```python
from build123d import *

# Parameters (mm, degrees)
SKETCH_W      = 100
SKETCH_H      = 80
SKETCH_R      = 1.75
PAD_DEPTH     = 4.5
CHAMFER_SIZE  = 1.5
SKETCH001_W   = 100
SKETCH001_H   = 80
SKETCH001_W_2 = 97
SKETCH001_H_2 = 77
PAD001_DEPTH  = 45
SKETCH002_W   = 100
SKETCH002_H   = 80
SKETCH002_R   = 1.75
PAD002_DEPTH  = 3.5


with BuildPart() as part:
    # Sketch → Pad (new body)
    with BuildSketch(Plane.XY):
        with Locations((-14.266246, -4.330319)):
            Rectangle(SKETCH_W, SKETCH_H)
        with Locations((-59.499317, 30.08403)):
            Circle(SKETCH_R, mode=Mode.SUBTRACT)
        with Locations((28.500683, 29.937424)):
            Circle(SKETCH_R, mode=Mode.SUBTRACT)
        with Locations((-59.584126, -34.915915)):
            Circle(SKETCH_R, mode=Mode.SUBTRACT)
        with Locations((28.415874, -35.062521)):
            Circle(SKETCH_R, mode=Mode.SUBTRACT)
    extrude(amount=PAD_DEPTH)

    # Chamfer
    chamfer_edges = [part.edges().sort_by_distance(p)[0] for p in [
        (-61.334126, -34.915915, 0),
        (26.665874, -35.062521, 0),
        (26.750683, 29.937424, 0),
        (-61.249317, 30.08403, 0),
    ]]
    chamfer(chamfer_edges, length=CHAMFER_SIZE)

    # Sketch001 (on Face3 of Chamfer) → Pad001 (join)
    with BuildSketch(Plane.XY.offset(4.5)):
        with Locations((-14.266246, -4.330319)):
            Rectangle(SKETCH001_W, SKETCH001_H)
        with Locations((-14.266246, -4.330319)):
            Rectangle(SKETCH001_W_2, SKETCH001_H_2, mode=Mode.SUBTRACT)
    extrude(amount=PAD001_DEPTH)

    # Sketch002 (on Face19 of Pad001) → Pad002 (join)
    with BuildSketch(Plane.XY.offset(49.5)):
        with Locations((-14.266246, -4.330319)):
            Rectangle(SKETCH002_W, SKETCH002_H)
        with Locations((-59.499317, 30.08403)):
            Circle(SKETCH002_R, mode=Mode.SUBTRACT)
        with Locations((-59.584126, -34.915915)):
            Circle(SKETCH002_R, mode=Mode.SUBTRACT)
        with Locations((28.500683, 29.937424)):
            Circle(SKETCH002_R, mode=Mode.SUBTRACT)
        with Locations((28.415874, -35.062521)):
            Circle(SKETCH002_R, mode=Mode.SUBTRACT)
    extrude(amount=PAD002_DEPTH)


solid = part.part
```
Here's how the part is built. I have some questions about the finished solid (model axes, mm). A direction names the side the tool comes from. Coordinates: 2 decimals unless noted, no trailing zeros. Order: outer loops, then holes, each group sorted by start corner. A loop starts at its lowest first (then second) coordinate and runs counter-clockwise, first axis right, second up.
1) Which directions (+Z, -Z, +X, -X, +Y, -Y) give clear straight access to the entire face, cutting with the end or side of a thin tool? Please do faces 1 (the face through (-61.332, -34.839, 51.226)), 2 (the face through (-15, -4, 4.5)).
2) Will these pins go through, and if not, where does the flat tip stop? pin 1 (4 mm diameter, centred on x = 28.5, y = 29.94, fed in from -Z); pin 2 (5.5 mm diameter, centred on x = 28.5, y = 29.94, fed in from -Z).
3) We'd pull the mould along Z, two halves only. Please class faces 3 (the face through (34.234, -5, 27)), 4 (the face through (-15, -4, 53)), 5 (the face through (-64.266, -5, 26)), 6 (the face through (-15, 34.17, 27)): +Z half, -Z half, draft (parallel to the pull), parting line (faces both ways), or undercut.
4) Imagine slicing it at C-C on x = 29. State how many separate pieces and enclosed holes the cut face has, and give its area (3 significant figures).
5) Imagine slicing it at B-B on z = 41. List the corners of the cut face in (x, y) for me, and give its area (3 significant figures).
6) I need wall thicknesses on line 1 (Y direction, x = 22.5, z = 10); line 2 (X direction, y = -38, z = 47.5); line 3 (Z direction, x = -54, y = 25). Which ranges of each line are inside material? Lowest first, please.
7) Imagine slicing it at A-A on x = 10. List the corners of the cut face in (y, z) for me, and give its area (3 significant figures).
Response values:
1. face 1: +Z, -Z
1. face 2: none
2. pin 1: stops at z = 1.25
2. pin 2: stops at z = 0.5
3. face 3: undercut
3. face 4: +Z half
3. face 5: draft
3. face 6: undercut
4. separate pieces: 4
4. enclosed holes: 0
4. area: 717 mm2
5. outline: (-64.27, -44.33) - (35.73, -44.33) - (35.73, 35.67) - (-64.27, 35.67) - close; hole (-62.77, -42.83) - (34.23, -42.83) - (34.23, 34.17) - (-62.77, 34.17) - close
5. area: 531 mm2
6. line 1: y = -44.33 to -42.83, 34.17 to 35.67
6. line 2: x = -64.27 to -62.77, 34.23 to 35.73
6. line 3: z = 0 to 4.5, 49.5 to 53
7. outline: (-44.33, 0) - (35.67, 0) - (35.67, 53) - (-44.33, 53) - close; hole (-42.83, 4.5) - (34.17, 4.5) - (34.17, 49.5) - (-42.83, 49.5) - close
7. area: 775 mm2
